The figure shows three views and two pictorial views of one solid part (mm, origin at its lowest corner). Answer the questions. A direction names the side the tool comes from. Coordinates: 2 decimals unless noted, no trailing zeros. Write each loop counter-clockwise with the first axis right and the second up, starting at its lowest first coordinate (ties: lowest second). Pieces come first, ordered by that corner, then holes. Notation, with made-up numbers: M 83,-6.5 L 126,-6.5 A18 cw 126,28.5 Z; hole C -37,-11 d9. An arc over 180 degrees is marked long. Write item = value, one per line. Start each with the question number.
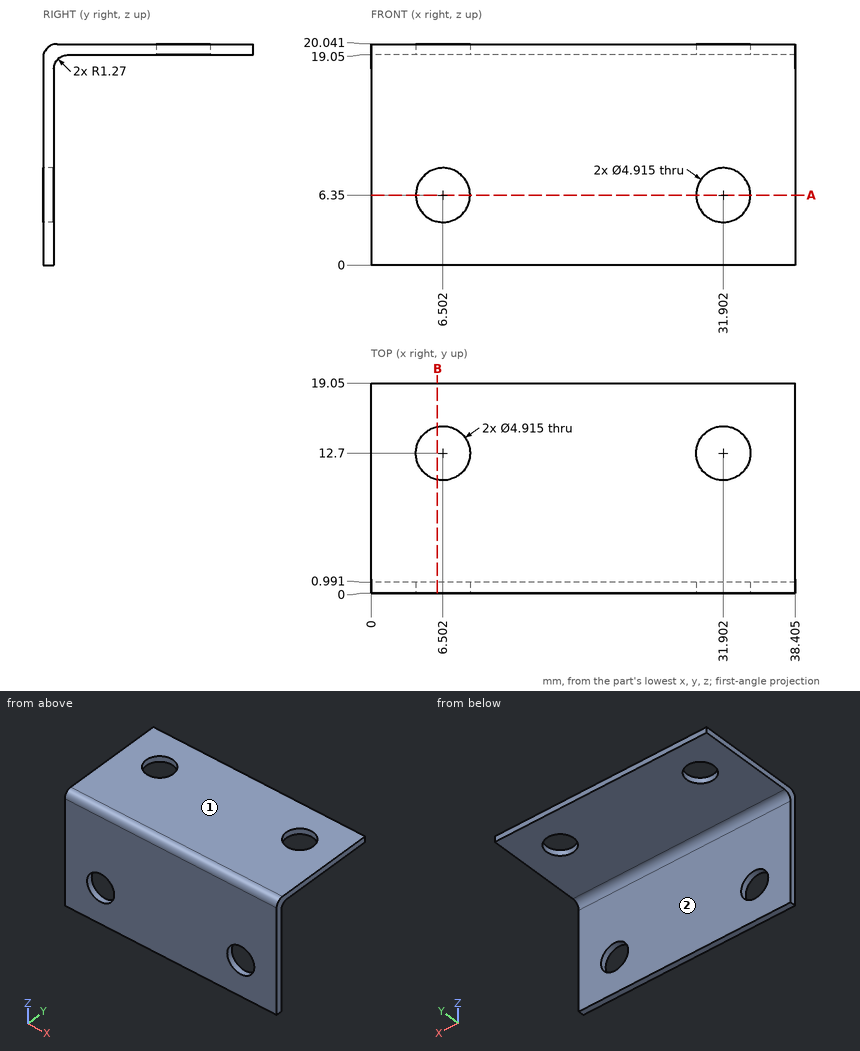
1. The part is cut by section B-B, the plane x = 6. Count the separate pieces of the cut face and the enclosed holes in it.
2. For the marked faces 1 and 2, determine the directions among +Z, -Z, +X, -X, +Y, -Y from which every point of the face is accessible in a straight line to the end or side of a thin tool.
3. Each of these flat-tipped pins is pushed along its axis until it touches: pin 1 (5 mm diameter, centred on x = 26, y = 14, fed in from -Z); pin 2 (5.5 mm diameter, centred on x = 11.5, z = 6.5, fed in from +Y); pin 3 (1 mm diameter, centred on x = 30.5, y = 2.5, fed in from -Z); pin 4 (4 mm diameter, centred on x = 31.9, z = 6.35, fed in from +Y). Where does it stop, or does it pass through?
4. Straight lines are drawn through the part: L1, parallel to Y at x = 3, z = 16.5; L2, parallel to Z at x = 7, y = 6.75; L3, parallel to Y at x = 2.5, z = 18.5 (1 decimal). For each, find the intervals that lie inside material, in ascending order. Write a range as [from, to].
5. The part is cut by section A-A, the plane z = 6.35. Write down the section's boundary in (x, y) (1 decimal).
Solution:
q1.separate_pieces = 3
q1.enclosed_holes = 0
q2.face_1 = +Z, +X, -X, +Y, -Y
q2.face_2 = -Z, +X, -X, +Y
q3.pin_1 = 19.05
q3.pin_2 = 0.99
q3.pin_3 = 19.02
q3.pin_4 = through
q4.L1 = [0, 0.99]
q4.L2 = [19.05, 20.04]
q4.L3 = [0, 1.2]
q5.outline = M 0,0 L 4,0 L 4,1 L 0,1 Z; M 9,0 L 29.4,0 L 29.4,1 L 9,1 Z; M 34.4,0 L 38.4,0 L 38.4,1 L 34.4,1 Z
